Part model, mm, in its own coordinate system. Face numbers are marked on the shaded views. A direction names the side the tool comes from. Round coordinates to 2 decimals unless told otherwise and drop trailing zeros. Loops run counter-clockwise (first coordinate to the right, second up) from the corner with the lowest first, then second, coordinate; pieces in that order, holes last. Notation, with made-up numbers: (-17, 40) -> (6, 40) arc R34 ccw to (6, 79) -> close; hole circle Ø1 at (67.5, 29). An arc over 180 degrees is marked (long way). Use a Markdown table: item, result. Add a question column.
Item 1: Cut at C-C, the plane x = 2.25. List the corners of the cut face in (y, z), plus the area to 3 significant figures.
Item 2: Cut at B-B, the plane y = 0. List the corners of the cut face in (x, z).
Item 3: Probe line 1 (Y direction, x = 1, z = 1.75); line 2 (Y direction, x = 18, z = -2.85); line 3 (Z direction, x = 12.25, y = -2.75). List the from-to ranges inside material, lowest first. Write a range as [from, to].
Item 4: Cut at A-A, the plane z = 1.5. List the corners of the cut face in (x, y).
Item 5: Cut at D-D, the plane x = 20.25. List the corners of the cut face in (y, z).
Item 6: Two-plate mould, pull along X, no slides. Class the marked faces 1, 2 and 3: pulls with the +X half, pulls with the -X half, needs draft (parallel to the pull), parting line crosses it, or undercut.
Item 7: Flat gauge pins, fed straight in: pin 1 (1 mm diameter, centred on x = 17, z = -2, fed in from -Y); pin 2 (1.5 mm diameter, centred on x = 12.5, y = -2.5, fed in from -Z); pin 3 (2.5 mm diameter, centred on x = 18, y = 1, fed in from -Z). Where does each tip first touch, or does it go through?
Item 8: Which spindle directions (+Z, -Z, +X, -X, +Y, -Y) get a long thin tool onto all of the face, cutting with end or side? Do the marked faces 4, 5 and 6. Say none if no direction does.
```python
from build123d import *
from build123d.topology import SkipClean

# Parameters (mm, degrees)
BOSS_EXTRU_1_DEPTH      = 4
ESQUISSE2_R             = 4
BOSS_EXTRU_2_DEPTH      = 6
ENL_V_START             = -6
ESQUISSE3_R             = 2.5
ENL_V_MAT_EXTRU_1_DEPTH = 5


with BuildPart() as part:
    # Esquisse1 → Boss.-Extru.1 (new body)
    with BuildSketch(Plane.XY):
        with BuildLine():
            Line((2, -3.5), (-2, -3.5))
            ThreePointArc((-2, -3.5), (-5.5, 0), (-2, 3.5))
            Line((-2, 3.5), (2, 3.5))
            Line((2, 3.5), (18, 4))
            ThreePointArc((18, 4), (22, 0), (18, -4))
            Line((18, -4), (2, -3.5))
        make_face()
        with BuildLine():
            Line((-2, 2.1), (2, 2.1))
            ThreePointArc((2, 2.1), (4.1, 0), (2, -2.1))
            Line((2, -2.1), (-2, -2.1))
            ThreePointArc((-2, -2.1), (-4.1, 0), (-2, 2.1))
        make_face(mode=Mode.SUBTRACT)
    extrude(amount=BOSS_EXTRU_1_DEPTH)

    # Esquisse2 → Boss.-Extru.2 (add)
    with SkipClean():  # the faces are left unmerged after this step: merging them gives an invalid solid
        with BuildSketch(Plane.XY):
            with Locations(Location((18, 0, 0), (0, 0, 266.420178784))):
                Circle(ESQUISSE2_R)
        extrude(amount=-BOSS_EXTRU_2_DEPTH)

    # Esquisse3 → Enlèv. mat.-Extru.1 (cut)
    with SkipClean():  # the faces are left unmerged after this step: merging them gives an invalid solid
        with BuildSketch(Plane.XY.offset(ENL_V_START)):
            with Locations((18, 0)):
                Circle(ESQUISSE3_R)
        extrude(amount=ENL_V_MAT_EXTRU_1_DEPTH, mode=Mode.SUBTRACT)


solid = part.part
```
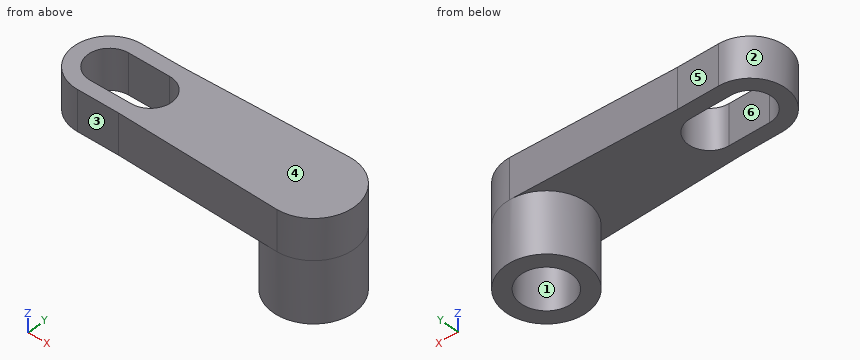
A:
| question | item | result |
|---|---|---|
| 1 | outline | (-3.51, 0) -> (-2.09, 0) -> (-2.09, 4) -> (-3.51, 4) -> close; (2.09, 0) -> (3.51, 0) -> (3.51, 4) -> (2.09, 4) -> close |
| 1 | area | 11.4 mm^2 |
| 2 | outline | (-5.5, 0) -> (-4.1, 0) -> (-4.1, 4) -> (-5.5, 4) -> close; (4.1, 0) -> (14, 0) -> (14, -6) -> (15.5, -6) -> (15.5, -1) -> (20.5, -1) -> (20.5, -6) -> (22, -6) -> (22, 4) -> (4.1, 4) -> close |
| 3 | line 1 | y = [-3.5, -2.1], [2.1, 3.5] |
| 3 | line 2 | y = [-4, -2.5], [2.5, 4] |
| 3 | line 3 | z = [0, 4] |
| 4 | outline | (-2, -3.5) -> (2, -3.5) -> (18, -4) arc R4 ccw to (18, 4) -> (2, 3.5) -> (-2, 3.5) arc R3.5 ccw to start; hole (-2, -2.1) -> (2, -2.1) arc R2.1 ccw to (2, 2.1) -> (-2, 2.1) arc R2.1 ccw to start |
| 5 | outline | (-3.31, -6) -> (-1.09, -6) -> (-1.09, -1) -> (1.09, -1) -> (1.09, -6) -> (3.31, -6) -> (3.31, 4) -> (-3.31, 4) -> close |
| 6 | face 1 | undercut |
| 6 | face 2 | pulls with the -X half |
| 6 | face 3 | needs draft |
| 7 | pin 1 | stops at y = -3.97 |
| 7 | pin 2 | stops at z = 0 |
| 7 | pin 3 | stops at z = -1 |
| 8 | face 4 | +Z, +X, -X, +Y, -Y |
| 8 | face 5 | +Z, -Z, -X, +Y |
| 8 | face 6 | +Z, -Z |
